Geometry: final body of the model. Coordinates: model frame, mm. A direction names the side the tool comes from. Give positions to 0.01 mm unless a question says otherwise; leave off trailing zeros. Loops run counter-clockwise (first coordinate to the right, second up) from the corner with the lowest first, then second, coordinate; pieces in that order, holes last.
1. Draft query along Z for faces 1 (the face through (6.89, 32.59, -20.43)), 2 (the face through (14.518, 50.089, 12.499)), 3 (the face through (-31.969, 51.511, -5.626)). Return one class per face: +Z half, -Z half, draft (parallel to the pull), parting line (faces both ways), or undercut.
2. Section B-B, the plane x = -25.4. Output: boundary loops of the cut face in (y, z), then the cut area to 3 significant figures.
3. First-contact query: P1, Ø5.5, axis at x = 0, y = 76.2, coming from the +Z side; P2, Ø1.8, axis at x = 6.35, y = 31.75, coming from the -Z side; P3, Ø3.5, axis at x = 26, y = 44.5, coming from the +Z side; P4, Ø1, axis at x = -24.5, y = 16.5, coming from the -Z side. Flat tips, straight axial feed; report the tip coordinate or a pass-through.
4. Access query for faces 4 (the face through (27, 50, 6.35)), 5 (the face through (-5.426, 5.967, -20.432)), 6 (the face through (-21.95, 51.51, -6.68)), 7 (the face through (-27, 50, 6.35)), 8 (the face through (14.4, 50.1, -12.7)). Directions: +Z, -Z, +X, -X, +Y, -Y. A direction counts if a zero-diameter tool reaches every point of the face in a straight line with its end or side. Return the directions, or none.
5. Section A-A, the plane x = 0. Output: boundary loops of the cut face in (y, z) (3 decimals).
6. Material intervals for line 1 along Y through (x, z) = (6.35, -19.75); line 2 along Z through (x, y) = (-25.4, 21); line 3 along Z through (x, y) = (-2, 45), sorted ascending.
7. Section C-C, the plane y = 76.2. State how many separate pieces and enclosed holes the cut face has, then the cut area to 3 significant figures.
from build123d import *

# Parameters (mm, degrees)
BOSS_EXTRUDE1_DEPTH = 101.6
FILLET1_R           = 2.54
SKETCH9_R           = 1
CUT_EXTRUDE7_DEPTH  = 3.175
SKETCH11_R          = 3.175
CUT_EXTRUDE8_DEPTH  = 44.994090512
SKETCH12_R          = 3.175
CUT_EXTRUDE9_DEPTH  = 62.34261314
SKETCH13_R          = 3.175
CUT_EXTRUDE10_DEPTH = 62.34261314


with BuildPart() as part:
    # Sketch2 → Boss-Extrude1 (new body)
    with BuildSketch(Plane(origin=(0, 0, 0), x_dir=(1, 0, 0), z_dir=(0, 1, 0))):
        with BuildLine():
            Line((-23.65375, 3.024593723), (-21.733825791, 6.35))
            Line((-21.733825791, 6.35), (-32.732348419, 6.35))
            Line((-32.732348419, 6.35), (-32.732348419, -6.35))
            Line((-32.732348419, -6.35), (-21.733825791, -6.35))
            Line((-21.733825791, -6.35), (-23.65375, -3.024593723))
            ThreePointArc((-23.65375, -3.024593723), (-28.8925, 0), (-23.65375, 3.024593723))
        make_face()
        with BuildLine():
            Line((32.732348419, 6.35), (21.733825791, 6.35))
            Line((21.733825791, 6.35), (23.65375, 3.024593723))
            ThreePointArc((23.65375, 3.024593723), (27.14625, 3.024593723), (28.8925, 0))
            ThreePointArc((28.8925, 0), (27.14625, -3.024593723), (23.65375, -3.024593723))
            Line((23.65375, -3.024593723), (21.733825791, -6.35))
            Line((21.733825791, -6.35), (32.732348419, -6.35))
            Line((32.732348419, -6.35), (32.732348419, 6.35))
        make_face()
        Polygon((12.7, 21.997045256), (-12.7, 21.997045256), (-21.733825791, 6.35), (-18.067651581, 6.35), (-10.866912895, 18.822045256), (10.866912895, 18.822045256), (18.067651581, 6.35), (21.733825791, 6.35), align=None)
        Polygon((-10.866912895, -18.822045256), (-18.067651581, -6.35), (-21.733825791, -6.35), (-12.7, -21.997045256), (12.7, -21.997045256), (21.733825791, -6.35), (18.067651581, -6.35), (10.866912895, -18.822045256), align=None)
        with BuildLine():
            Line((-18.067651581, 6.35), (-21.733825791, 6.35))
            Line((-21.733825791, 6.35), (-23.65375, 3.024593723))
            ThreePointArc((-23.65375, 3.024593723), (-22.375406277, 1.74625), (-21.9075, 0))
            ThreePointArc((-21.9075, 0), (-22.375406277, -1.74625), (-23.65375, -3.024593723))
            Line((-23.65375, -3.024593723), (-21.733825791, -6.35))
            Line((-21.733825791, -6.35), (-18.067651581, -6.35))
            Line((-18.067651581, -6.35), (-21.733825791, 0))
            Line((-21.733825791, 0), (-18.067651581, 6.35))
        make_face()
        Polygon((-18.067651581, -6.35), (-18.067651581, 6.35), (-21.733825791, 0), align=None)
        with BuildLine():
            Line((23.65375, 3.024593723), (21.733825791, 6.35))
            Line((21.733825791, 6.35), (18.067651581, 6.35))
            Line((18.067651581, 6.35), (21.733825791, 0))
            Line((21.733825791, 0), (18.067651581, -6.35))
            Line((18.067651581, -6.35), (21.733825791, -6.35))
            Line((21.733825791, -6.35), (23.65375, -3.024593723))
            ThreePointArc((23.65375, -3.024593723), (21.9075, 0), (23.65375, 3.024593723))
        make_face()
        Polygon((21.733825791, 0), (18.067651581, 6.35), (18.067651581, -6.35), align=None)
    extrude(amount=BOSS_EXTRUDE1_DEPTH)

    # Fillet1
    fillet1_edges = [part.edges().sort_by_distance(p)[0] for p in [
        (21.733825791, 50.8, -6.35),
        (32.732348419, 50.8, -6.35),
        (32.732348419, 50.8, 6.35),
        (21.733825791, 50.8, 6.35),
        (-21.733825791, 50.8, 6.35),
        (-32.732348419, 50.8, 6.35),
        (-32.732348419, 50.8, -6.35),
        (-21.733825791, 50.8, -6.35),
    ]]
    fillet(fillet1_edges, radius=FILLET1_R)

    # Sketch9 → Cut-Extrude7 (cut)
    with BuildSketch(Plane.XY.offset(-21.997045256)):
        with Locations((-6.35, 6.35)):
            Circle(SKETCH9_R)
        with Locations((-6.35, 24.13)):
            Circle(SKETCH9_R)
        with Locations((6.35, 6.35)):
            Circle(SKETCH9_R)
        with Locations((6.35, 24.13)):
            Circle(SKETCH9_R)
        with Locations((-6.35, 49.53)):
            Circle(SKETCH9_R)
        with Locations((-6.35, 31.75)):
            Circle(SKETCH9_R)
        with Locations((6.35, 49.53)):
            Circle(SKETCH9_R)
        with Locations((6.35, 31.75)):
            Circle(SKETCH9_R)
    extrude(amount=CUT_EXTRUDE7_DEPTH, mode=Mode.SUBTRACT)

    # Sketch11 → Cut-Extrude8 (cut, through all)
    with BuildSketch(Plane(origin=(0, 0, -21.997045256), x_dir=(-1, 0, 0), z_dir=(0, 0, -1))):
        with Locations((0, 76.2)):
            Circle(SKETCH11_R)
    extrude(amount=-CUT_EXTRUDE8_DEPTH, mode=Mode.SUBTRACT)

    # Sketch12 → Cut-Extrude9 (cut, through all)
    with BuildSketch(Plane(origin=(-19.05, 0, -10.998522628), x_dir=(-0.5, 0, 0.866025404), z_dir=(-0.866025404, 0, -0.5))):
        with Locations((0, 63.5)):
            Circle(SKETCH12_R)
    extrude(amount=-CUT_EXTRUDE9_DEPTH, mode=Mode.SUBTRACT)

    # Sketch13 → Cut-Extrude10 (cut, through all)
    with BuildSketch(Plane(origin=(19.05, 0, -10.998522628), x_dir=(-0.5, 0, -0.866025404), z_dir=(0.866025404, 0, -0.5))):
        with Locations((0, 50.8)):
            Circle(SKETCH13_R)
    extrude(amount=-CUT_EXTRUDE10_DEPTH, mode=Mode.SUBTRACT)


solid = part.part
Answers below:
1. face 1: draft
1. face 2: undercut
1. face 3: -Z half
2. outline: (0, -6.35) - (101.6, -6.35) - (101.6, -3.49) - (0, -3.49) - close; (0, 3.49) - (101.6, 3.49) - (101.6, 6.35) - (0, 6.35) - close
2. area: 581 mm2
3. P1: passes through
3. P2: stops at z = 18.82
3. P3: stops at z = 6.35
3. P4: stops at z = -6.35
4. face 4: +Z, +X, +Y, -Y
4. face 5: -Z
4. face 6: -Z, -X, +Y, -Y
4. face 7: +Z, -X, +Y, -Y
4. face 8: +Y, -Y
5. outline: (0, -21.997) - (73.025, -21.997) - (73.025, -18.822) - (0, -18.822) - close; (0, 18.822) - (73.025, 18.822) - (73.025, 21.997) - (0, 21.997) - close; (79.375, -21.997) - (101.6, -21.997) - (101.6, -18.822) - (79.375, -18.822) - close; (79.375, 18.822) - (101.6, 18.822) - (101.6, 21.997) - (79.375, 21.997) - close
6. line 1: y = 0 to 5.35, 7.35 to 23.13, 25.13 to 30.75, 32.75 to 48.53, 50.53 to 101.6
6. line 2: z = -6.35 to -3.49, 3.49 to 6.35
6. line 3: z = -22 to -18.82, 18.82 to 22
7. separate pieces: 2
7. enclosed holes: 2
7. area: 607 mm2
